The model under review builds one solid part; all positions refer to its coordinate system, in mm. A direction names the side the tool comes from. Coordinates: 2 decimals unless noted, no trailing zeros. Write each loop counter-clockwise with the first axis right and the second up, starting at its lowest first coordinate (ties: lowest second). Pieces come first, ordered by that corner, then holes.
```python
from build123d import *

# Parameters (mm, degrees)
RESSALTO_EXTRUS_O1_DEPTH = 18
CORTE_EXTRUS_O1_DEPTH    = 16
ESBO_O3_R                = 1.5
CORTE_EXTRUS_O2_DEPTH    = 16
ESBO_O4_R                = 1.5
CORTE_EXTRUS_O5_DEPTH    = 5
ESBO_O11_R               = 1.5
CORTE_EXTRUS_O6_DEPTH    = 5
ESBO_O16_R               = 2
CORTE_EXTRUS_O7_DEPTH    = 5
ESBO_O17_R               = 1.25
CORTE_EXTRUS_O8_DEPTH    = 10
FILETE1_R                = 5
FILETE2_R                = 5
FILETE3_R                = 5
FILETE4_R                = 5
FILETE5_R                = 5
FILETE6_R                = 5
FILETE7_R                = 5
FILETE8_R                = 5


with BuildPart() as part:
    # Esboço1 → Ressalto-extrusão1 (new body)
    with BuildSketch(Plane(origin=(0, 0, 0), x_dir=(1, 0, 0), z_dir=(0, 1, 0))):
        with BuildLine():
            ThreePointArc((-20.749133867, -1.000866133), (-21.131951371, -0.000598593), (-20.75, 1))
            Line((-20.75, 1), (-11, 10.75))
            Line((-11, 10.75), (11, 10.75))
            Line((11, 10.75), (20.75, 1))
            ThreePointArc((20.75, 1), (21.131966011, 0), (20.750111133, -0.999888867))
            Line((20.750111133, -0.999888867), (11, -10.75))
            Line((11, -10.75), (-11, -10.75))
            Line((-11, -10.75), (-20.749133867, -1.000866133))
        make_face()
    extrude(amount=RESSALTO_EXTRUS_O1_DEPTH)

    # Esboço2 → Corte-extrusão1 (cut)
    with BuildSketch(Plane(origin=(0, 18, 0), x_dir=(1, 0, 0), z_dir=(0, 1, 0))):
        with BuildLine():
            Line((9.972089297, 9.55), (-10.502943725, 9.55))
            Line((-10.502943725, 9.55), (-19.052943725, 1))
            Line((-19.052943725, 1), (-19.389618767, 0.663324958))
            ThreePointArc((-19.389618767, 0.663324958), (-19.589618767, 0), (-19.389618767, -0.663324958))
            Line((-19.389618767, -0.663324958), (-19.052943725, -1))
            Line((-19.052943725, -1), (-10.502943725, -9.55))
            Line((-10.502943725, -9.55), (10.502943725, -9.55))
            Line((10.502943725, -9.55), (19.052943725, -1))
            ThreePointArc((19.052943725, -1), (19.434909736, 0), (19.052943725, 1))
            Line((19.052943725, 1), (11.538307765, 8.51463596))
            Line((11.538307765, 8.51463596), (10.502943725, 9.55))
            Line((10.502943725, 9.55), (9.972089297, 9.55))
        make_face()
    extrude(amount=-CORTE_EXTRUS_O1_DEPTH, mode=Mode.SUBTRACT)

    # Esboço3 → Corte-extrusão2 (cut)
    with BuildSketch(Plane(origin=(0, 0, 9.55), x_dir=(-1, 0, 0), z_dir=(0, 0, -1))):
        with Locations((0, 8)):
            Circle(ESBO_O3_R)
    extrude(amount=-CORTE_EXTRUS_O2_DEPTH, mode=Mode.SUBTRACT)

    # Esboço4 → Corte-extrusão5 (cut)
    with BuildSketch(Plane(origin=(10.026471863, 0, 10.026471863), x_dir=(-0.7071067811865475, 0, 0.7071067811865477), z_dir=(-0.7071067811865477, 0, -0.7071067811865475))):
        with Locations((-4.67383297, 8)):
            Circle(ESBO_O4_R)
    extrude(amount=-CORTE_EXTRUS_O5_DEPTH, mode=Mode.SUBTRACT)

    # Esboço11 → Corte-extrusão6 (cut)
    with BuildSketch(Plane(origin=(-10.026471863, 0, 10.026471863), x_dir=(-0.7071067811865477, 0, -0.7071067811865474), z_dir=(0.7071067811865474, 0, -0.7071067811865477))):
        with Locations((4.67383297, 8)):
            Circle(ESBO_O11_R)
    extrude(amount=-CORTE_EXTRUS_O6_DEPTH, mode=Mode.SUBTRACT)

    # Esboço16 → Corte-extrusão7 (cut)
    with BuildSketch(Plane(origin=(0, 2, 0), x_dir=(1, 0, 0), z_dir=(0, 1, 0))):
        with Locations(Location((-9.75, 0.45, 0), (0, 0, 270))):
            Circle(ESBO_O16_R)
        with Locations(Location((9.75, 0.45, 0), (0, 0, 270))):
            Circle(ESBO_O16_R)
        with Locations(Location((0, 3.45, 0), (0, 0, 270))):
            Circle(ESBO_O16_R)
    extrude(amount=-CORTE_EXTRUS_O7_DEPTH, mode=Mode.SUBTRACT)

    # Esboço17 → Corte-extrusão8 (cut)
    with BuildSketch(Plane(origin=(0, 2, 0), x_dir=(1, 0, 0), z_dir=(0, 1, 0))):
        with Locations(Location((-6, -6.55, 0), (0, 0, 270))):
            Circle(ESBO_O17_R)
        with Locations(Location((6, -6.55, 0), (0, 0, 270))):
            Circle(ESBO_O17_R)
    extrude(amount=-CORTE_EXTRUS_O8_DEPTH, mode=Mode.SUBTRACT)

    # Filete1
    filete1_edges = [part.edges().sort_by_distance(p)[0] for p in [
        (-10.502943725, 10, -9.55),
    ]]
    fillet(filete1_edges, radius=FILETE1_R)

    # Filete2
    filete2_edges = [part.edges().sort_by_distance(p)[0] for p in [
        (10.502943725, 10, -9.55),
    ]]
    fillet(filete2_edges, radius=FILETE2_R)

    # Filete3
    filete3_edges = [part.edges().sort_by_distance(p)[0] for p in [
        (-10.502943725, 10, 9.55),
    ]]
    fillet(filete3_edges, radius=FILETE3_R)

    # Filete4
    filete4_edges = [part.edges().sort_by_distance(p)[0] for p in [
        (10.502943725, 10, 9.55),
    ]]
    fillet(filete4_edges, radius=FILETE4_R)

    # Filete5
    filete5_edges = [part.edges().sort_by_distance(p)[0] for p in [
        (-11, 9, -10.75),
    ]]
    fillet(filete5_edges, radius=FILETE5_R)

    # Filete6
    filete6_edges = [part.edges().sort_by_distance(p)[0] for p in [
        (11, 9, -10.75),
    ]]
    fillet(filete6_edges, radius=FILETE6_R)

    # Filete7
    filete7_edges = [part.edges().sort_by_distance(p)[0] for p in [
        (-11, 9, 10.75),
    ]]
    fillet(filete7_edges, radius=FILETE7_R)

    # Filete8
    filete8_edges = [part.edges().sort_by_distance(p)[0] for p in [
        (11, 9, 10.75),
    ]]
    fillet(filete8_edges, radius=FILETE8_R)


solid = part.part
```
Item 1: Mouldability with a two-part tool opening along X and no side actions: class faces 3 (the face through (0, 9, -10.75)), 4 (the face through (-10.87, 9.13, 10.36)), 5 (the face through (0.325, 6.536, 10.142)) as pulls with the +X half, pulls with the -X half, needs draft (parallel to the pull), parting line crosses it, or undercut.
Solved:
face 3: needs draft
face 4: pulls with the -X half
face 5: undercut
Item 2: Machinability: for faces 1 (the face through (-10.32, 9.89, -9.18)), 2 (the face through (-0.766, 1.014, -1.603)), which of the approach directions +Z, -Z, +X, -X, +Y, -Y give a long, thin tool a straight path to every point of the face, cutting with its end or side? Answer none if there is none.
Solved:
face 1: +Y
face 2: +Y, -Y
Item 3: Take a section at B-B, the plane y = 16.75. Write out the cut boundary in (x, z).
Solved:
outline: (-20.75, -1) - (-12.46, -9.29) arc R5 ccw to (-8.93, -10.75) - (8.93, -10.75) arc R5 ccw to (12.46, -9.29) - (20.75, -1) arc R1.5 ccw to (20.75, 1) - (12.46, 9.29) arc R5 ccw to (8.93, 10.75) - (-8.93, 10.75) arc R5 ccw to (-12.46, 9.29) - (-20.75, 1) arc R1.5 ccw to start; hole (-19.39, -0.66) - (-11.97, -8.09) arc R5 ccw to (-8.43, -9.55) - (8.43, -9.55) arc R5 ccw to (11.97, -8.09) - (19.05, -1) arc R1.5 ccw to (19.05, 1) - (11.97, 8.09) arc R5 ccw to (8.43, 9.55) - (-8.43, 9.55) arc R5 ccw to (-11.97, 8.09) - (-19.39, 0.66) arc R1.2 ccw to start
Item 4: For pin 1 (1.5 mm diameter, centred on x = 1, z = 4, fed in from +Y); pin 2 (3.5 mm diameter, centred on x = 9.75, z = -0.45, fed in from -Y); pin 3 (2 mm diameter, centred on x = -10.5, y = 3, fed in from -Z), all flat-tipped, find the tip position at first contact; note any pin that passes through.
Solved:
pin 1: stops at y = 2
pin 2: passes through
pin 3: stops at z = -10.72
Item 5: Take a section at C-C, the plane z = 0.25. Write out the cut boundary in (x, y), plus the area to 3 significant figures.
Solved:
outline: (-21.11, 0) - (-11.62, 0) - (-11.62, 2) - (-19.56, 2) - (-19.56, 18) - (-21.11, 18) - close; (-7.88, 0) - (7.88, 0) - (7.88, 2) - (-7.88, 2) - close; (11.62, 0) - (21.11, 0) - (21.11, 18) - (19.41, 18) - (19.41, 2) - (11.62, 2) - close
area: 121 mm2
Item 6: Take a section at D-D, the plane x = 6. Write out the cut boundary in (y, z), plus the area to 3 significant figures.
Solved:
outline: (0, -10.75) - (18, -10.75) - (18, -9.55) - (2, -9.55) - (2, 5.3) - (0, 5.3) - close; (0, 7.8) - (2, 7.8) - (2, 9.55) - (18, 9.55) - (18, 10.75) - (0, 10.75) - close
area: 76.4 mm2
Item 7: To check wall thickness, follow line 1 along X through (y, z) = (1.55, 6.55); line 2 along Z through (x, y) = (5, 7.5); line 3 along Z through (x, y) = (14, 5.25). State the ranges of each line that lie inside material, in increasing order.
Solved:
line 1: x = -15.2 to -7.25, -4.75 to 4.75, 7.25 to 15.2
line 2: z = -10.75 to -9.55, 9.55 to 10.75
line 3: z = -7.75 to -6.05, 6.05 to 7.75
Item 8: Take a section at A-A, the plane x = 0. Write out the cut boundary in (y, z).
Solved:
outline: (0, -10.75) - (18, -10.75) - (18, -9.55) - (2, -9.55) - (2, -5.45) - (0, -5.45) - close; (0, -1.45) - (2, -1.45) - (2, 9.55) - (6.5, 9.55) - (6.5, 10.75) - (0, 10.75) - close; (9.5, 9.55) - (18, 9.55) - (18, 10.75) - (9.5, 10.75) - close
